Could you check a few things on this model? Use its own coordinates, in mm. Face numbers are marked on the shaded views. Give positions to 0.01 mm unless a question says otherwise; leave off trailing zeros. Order: outer loops, then holes, each group sorted by start corner. A loop starts at its lowest first (then second) coordinate and runs counter-clockwise, first axis right, second up. Notation, with made-up numbers: (-23.75, 45.25) -> (26.25, 45.25) arc R4 cw to (26.25, 50.25) -> close; hole circle Ø4 at (87.25, -9.75). An arc over 180 degrees is marked (long way). Use one line per item in the form item = value. Start each with the question number.
from build123d import *

# Parameters (mm, degrees)
SKETCH1_R           = 1.5
BOSS_EXTRUDE1_DEPTH = 2.5


with BuildPart() as part:
    # Sketch1 → Boss-Extrude1 (new body, symmetric)
    with BuildSketch(Plane(origin=(0, 0, 0), x_dir=(0, 0, -1), z_dir=(1, 0, 0))):
        with BuildLine():
            Line((23.3, 18.1), (35.3, 2.1))
            ThreePointArc((35.3, 2.1), (34.6, -2.8), (29.7, -2.1))
            Line((29.7, -2.1), (17.7, 13.9))
            ThreePointArc((17.7, 13.9), (15.406888371, 15.813776741), (12.5, 16.5))
            Line((12.5, 16.5), (-12.5, 16.5))
            ThreePointArc((-12.5, 16.5), (-15.406888371, 15.813776741), (-17.7, 13.9))
            Line((-17.7, 13.9), (-29.7, -2.1))
            ThreePointArc((-29.7, -2.1), (-34.6, -2.8), (-35.3, 2.1))
            Line((-35.3, 2.1), (-23.3, 18.1))
            ThreePointArc((-23.3, 18.1), (-18.537383539, 22.074767078), (-12.5, 23.5))
            Line((-12.5, 23.5), (12.5, 23.5))
            ThreePointArc((12.5, 23.5), (18.537383539, 22.074767078), (23.3, 18.1))
        make_face()
        with Locations((-32.5, 0)):
            Circle(SKETCH1_R, mode=Mode.SUBTRACT)
        with Locations((32.5, 0)):
            Circle(SKETCH1_R, mode=Mode.SUBTRACT)
        with Locations((0, 20)):
            Circle(SKETCH1_R, mode=Mode.SUBTRACT)
    extrude(amount=BOSS_EXTRUDE1_DEPTH, both=True)


solid = part.part
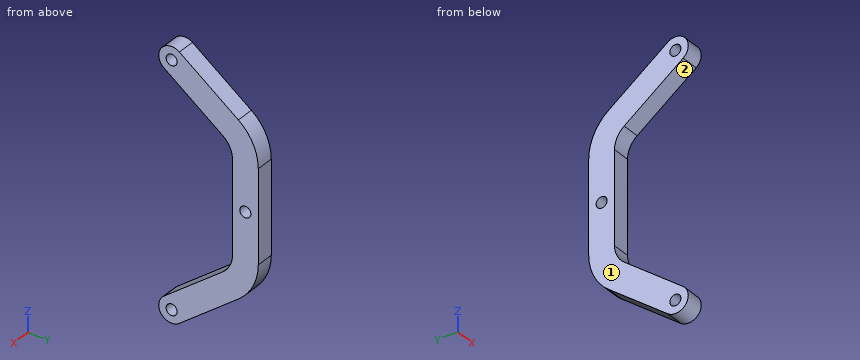
(1) I'm going to push flat-ended pins straight in: pin 1 Ø3 at (x, y) = (1.5, 9.5) entering from +Z (3 decimals); pin 2 Ø1.5 at (x, z) = (2, -28.5) entering from -Y. Where does each tip first touch, or does it pass through?
(2) Please list where these lines run through material, in increasing order: probe 1 along Z at (x, y) = (1.95, 1.75); probe 2 along Y at (x, z) = (-0.95, 7); probe 3 along Y at (x, z) = (1.3, -32.5).
(3) Imagine slicing it at D-D (z = -32.5). Write out the boundary of the cut face in (x, y).
(4) Imagine slicing it at B-B (x = 1.7). Write out the boundary of the cut face in (y, z).
(5) We'd pull the mould along Z, two halves only. Please class the marked faces 1 and 2: pulls with the +Z half, pulls with the -Z half, needs draft (parallel to the pull), parting line crosses it, or undercut.
(6) Imagine slicing it at C-C (y = 0). Write out the boundary of the cut face in (x, z) (3 decimals), plus the area to 4 significant figures.
(7) Imagine slicing it at A-A (y = 11.5). Write out the boundary of the cut face in (x, z).
Calculated:
q1.pin_1 = 30.875
q1.pin_2 = -1.5
q2.probe_1 = -35.53 to -26.81, 26.81 to 35.53
q2.probe_2 = 16.5 to 23.5
q2.probe_3 = -3.5 to -1.5, 1.5 to 5.83
q3.outline = (-2.5, -3.5) -> (2.5, -3.5) -> (2.5, -1.5) -> (-2.5, -1.5) -> close; (-2.5, 1.5) -> (2.5, 1.5) -> (2.5, 5.83) -> (-2.5, 5.83) -> close
q4.outline = (-2.1, -29.7) arc R3.5 ccw to (2.1, -35.3) -> (18.1, -23.3) arc R13.5 ccw to (23.5, -12.5) -> (23.5, 12.5) arc R13.5 ccw to (18.1, 23.3) -> (2.1, 35.3) arc R3.5 ccw to (-2.1, 29.7) -> (13.9, 17.7) arc R6.5 cw to (16.5, 12.5) -> (16.5, -12.5) arc R6.5 cw to (13.9, -17.7) -> close; hole circle Ø3 at (0, -32.5); hole circle Ø3 at (0, 32.5); hole circle Ø3 at (20, 0)
q5.face_1 = needs draft
q5.face_2 = undercut
q6.outline = (-2.5, -36) -> (2.5, -36) -> (2.5, -34) -> (-2.5, -34) -> close; (-2.5, -31) -> (2.5, -31) -> (2.5, -28.125) -> (-2.5, -28.125) -> close; (-2.5, 28.125) -> (2.5, 28.125) -> (2.5, 31) -> (-2.5, 31) -> close; (-2.5, 34) -> (2.5, 34) -> (2.5, 36) -> (-2.5, 36) -> close
q6.area = 48.75 mm2
q7.outline = (-2.5, -28.25) -> (2.5, -28.25) -> (2.5, -19.5) -> (-2.5, -19.5) -> close; (-2.5, 19.5) -> (2.5, 19.5) -> (2.5, 28.25) -> (-2.5, 28.25) -> close
